from build123d import *

# Parameters (mm, degrees)
BOSS_EXTRUDE1_DEPTH = 10
CUT_EXTRUDE1_DEPTH  = 61


with BuildPart() as part:
    # Sketch2 → Boss-Extrude1 (new body)
    with BuildSketch(Plane.XY):
        Polygon((-60, 30), (-95, 30), (-95, -30), (95, -30), (95, 30), (0, 30), (0, -5), (-60, -5), align=None)
    extrude(amount=BOSS_EXTRUDE1_DEPTH)

    # Sketch3 → Cut-Extrude1 (cut, through all)
    with BuildSketch(Plane(origin=(0, 30, 0), x_dir=(1, 0, 0), z_dir=(0, 1, 0))):
        with BuildLine():
            ThreePointArc((-78.975, -5), (-77.5, -6.475), (-76.025, -5))
            Line((-76.025, -5), (-78.975, -5))
        make_face()
        with BuildLine():
            Line((-78.975, -5), (-76.025, -5))
            ThreePointArc((-76.025, -5), (-77.5, -3.525), (-78.975, -5))
        make_face()
        with BuildLine():
            ThreePointArc((58.525, -5), (60, -6.475), (61.475, -5))
            Line((61.475, -5), (58.525, -5))
        make_face()
        with BuildLine():
            Line((58.525, -5), (61.475, -5))
            ThreePointArc((61.475, -5), (60, -3.525), (58.525, -5))
        make_face()
        with BuildLine():
            ThreePointArc((23.525, -5), (25, -6.475), (26.475, -5))
            Line((26.475, -5), (23.525, -5))
        make_face()
        with BuildLine():
            Line((23.525, -5), (26.475, -5))
            ThreePointArc((26.475, -5), (25, -3.525), (23.525, -5))
        make_face()
    extrude(amount=-CUT_EXTRUDE1_DEPTH, mode=Mode.SUBTRACT)


solid = part.part
Could you check a few things on this model? Use its own coordinates, in mm. A direction names the side the tool comes from. Give positions to 0.01 mm unless a question says otherwise; leave off trailing zeros. Loops run counter-clockwise (first coordinate to the right, second up) from the corner with the lowest first, then second, coordinate; pieces in that order, holes last. Notation, with made-up numbers: (-34, 31) -> (3, 31) arc R16 ccw to (3, 47) -> close; hole circle Ø6 at (88.5, 61). An arc over 180 degrees is marked (long way). Answer as CSV lines item,"result". Start each with the question number.
(1) I need wall thicknesses on probe 1 along X at (y, z) = (-13.5, 5) (3 decimals); probe 2 along X at (y, z) = (-3.5, 5) (3 decimals); probe 3 along Z at (x, y) = (25, -15.5) (3 decimals). Which ranges of each line are inside material? Lowest first, please.
(2) If we section it at A-A on y = 6: Write out the boundary of the cut face in (x, z) (3 decimals), then the cut area to 3 significant figures.
(3) Which directions (+Z, -Z, +X, -X, +Y, -Y) give clear straight access to the entire face, cutting with the end or side of a thin tool? Please do faces 1 (the flat face through (-60, 12, 5)), 2 (the flat face through (-1, -6, 10)).
(4) If we section it at B-B on z = 1.5: Write out the boundary of the cut face in (x, y).
(5) I'm going to push flat-ended pins straight in: pin 1 Ø2.5 at (x, z) = (25, 5) entering from -Y; pin 2 Ø1 at (x, z) = (-45.5, 1.5) entering from +Y. Where does each tip first touch, or does it pass through?
(6) We'd pull the mould along X, two halves only. Please class faces 3 (the flat face through (95, 0, 5)), 4 (the flat face through (-95, 0, 5)), 5 (the flat face through (-30, -5, 5)), 6 (the flat face through (0, 13, 5)): released by +X, released by -X, zero draft, split by the parting line, or undercut.
Computed:
1,probe 1,"x = -95 to -78.975, -76.025 to 23.525, 26.475 to 58.525, 61.475 to 95"
1,probe 2,"x = -95 to -78.975, -76.025 to -60, 0 to 23.525, 26.475 to 58.525, 61.475 to 95"
1,probe 3,"z = 0 to 3.525, 6.475 to 10"
2,outline,"(-95, 0) -> (-60, 0) -> (-60, 10) -> (-95, 10) -> close; (0, 0) -> (95, 0) -> (95, 10) -> (0, 10) -> close; hole circle Ø2.95 at (-77.5, 5); hole circle Ø2.95 at (25, 5); hole circle Ø2.95 at (60, 5)"
2,area,"1,280 mm2"
3,face 1,"+Z, -Z, +Y"
3,face 2,"+Z, +X, -X, +Y, -Y"
4,outline,"(-95, -30) -> (95, -30) -> (95, 30) -> (0, 30) -> (0, -5) -> (-60, -5) -> (-60, 30) -> (-95, 30) -> close"
5,pin 1,"passes through"
5,pin 2,"stops at y = -5"
6,face 3,"released by +X"
6,face 4,"released by -X"
6,face 5,"undercut"
6,face 6,"undercut"
